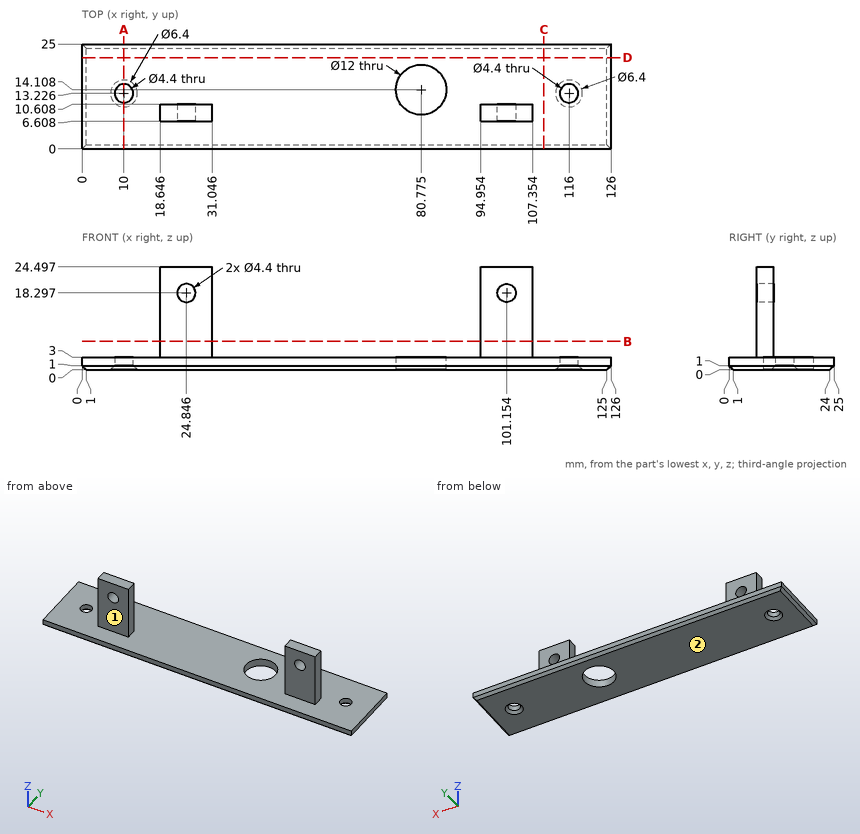
Input: dimensioned drawing with shaded views. Units: mm. Origin: part minimum x, y, z. Give positions to 0.01 mm unless a question says otherwise; leave off trailing zeros. Loops run counter-clockwise (first coordinate to the right, second up) from the corner with the lowest first, then second, coordinate; pieces in that order, holes last. Notation, with made-up numbers: M 72,-37 L 83,-37 A20 cw 83,-27 Z; hole C -37,85.5 d1. An arc over 180 degrees is marked long. Put each result on its own line as item: value.
1) Cut plane B-B, the plane z = 6.75. Return the cut outline in (x, y), plus the area to 3 significant figures.
Computed values:
outline: M 18.65,6.61 L 31.05,6.61 L 31.05,10.61 L 18.65,10.61 Z; M 94.95,6.61 L 107.35,6.61 L 107.35,10.61 L 94.95,10.61 Z
area: 99.2 mm^2
2) Cut plane C-C, the plane x = 110. Return the cut outline in (y, z), plus the area to 3 significant figures.
Computed values:
outline: M 0,1 L 1,0 L 24,0 L 25,1 L 25,3 L 0,3 Z
area: 74.0 mm^2
3) Mould query, pull axis Z, two halves, no side actions, for the marked faces 1 and 2. Classes: released by +Z, released by -Z, zero draft, split by the parting line, or undercut.
Computed values:
face 1: zero draft
face 2: released by -Z
4) First-contact query: P1, Ø13.5, axis at x = 22, z = 10.5, coming from the +Y side; P2, Ø8, axis at y = 14.5, z = 16, coming from the +X side; P3, Ø2, axis at y = 7.5, z = 8.5, coming from the -X side; P4, Ø12, axis at x = 44.5, z = 5, coming from the +Y side. Flat tips, straight axial feed; report the tip coordinate or a pass-through.
Computed values:
P1: stops at y = 10.61
P2: stops at x = 107.35
P3: stops at x = 18.65
P4: stops at y = 25
5) Cut plane A-A, the plane x = 10. Return the cut outline in (y, z), plus the area to 3 significant figures.
Computed values:
outline: M 0,1 L 1,0 L 10.03,0 L 11.03,1 L 11.03,3 L 0,3 Z; M 15.43,1 L 16.43,0 L 24,0 L 25,1 L 25,3 L 15.43,3 Z
area: 59.8 mm^2
6) Material intervals for L1, parallel to X at y = 9.5, z = 9.5; L2, parallel to Z at x = 48.5, y = 1.5; L3, parallel to Y at x = 30, z = 8.5, sorted ascending. Write a range as from..to.
Computed values:
L1: x = 18.65..31.05, 94.95..107.35
L2: z = 0..3
L3: y = 6.61..10.61
7) Cut plane D-D, the plane y = 21.75. Return the cut outline in (x, z), plus the area to 3 significant figures.
Computed values:
outline: M 0,1 L 1,0 L 125,0 L 126,1 L 126,3 L 0,3 Z
area: 377 mm^2
